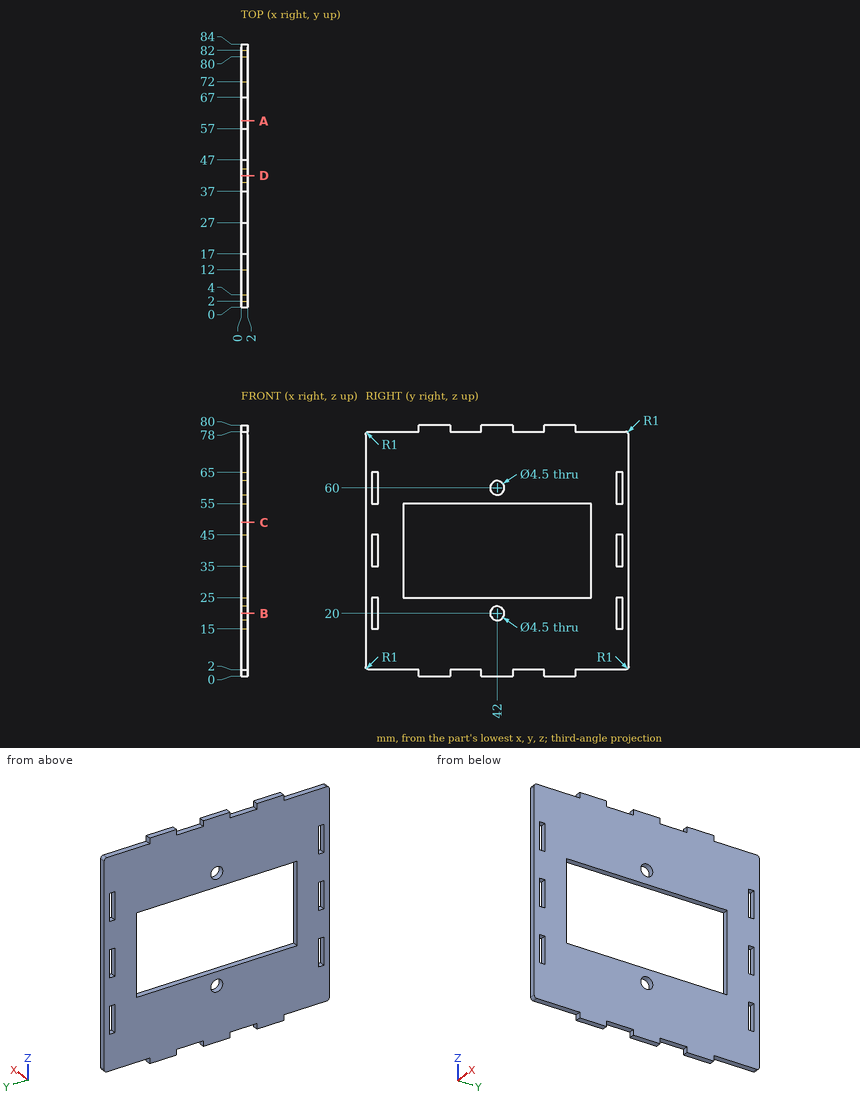
Drawing for the job (mm, zero at the part's lowest x, y, z). Round coordinates to 2 decimals unless told otherwise and drop trailing zeros. Loops run counter-clockwise (first coordinate to the right, second up) from the corner with the lowest first, then second, coordinate; pieces in that order, holes last. Notation, with made-up numbers: (37.25, 65) -> (79.25, 65) arc R16 cw to (79.25, 80) -> close; hole circle Ø4 at (-40, 6). An arc over 180 degrees is marked (long way). Use one line per item in the form item = value. Start each with the question number.
Item 1: Drop flat-ended pins along their axis: pin 1 Ø0.6 at (x, z) = (0.5, 79) entering from -Y; pin 2 Ø1 at (x, z) = (1, 1) entering from +Y. Give the stop position or say it passes through.
Item 2: Band-saw the part on D-D (y = 42). List the corners of the cut face in (x, z), plus the area to 3 significant figures.
Item 3: Drill centre lines: line 1 along Y through (x, z) = (1.4, 62.5); line 2 along Z through (x, y) = (1.5, 42); line 3 along Z through (x, y) = (1.05, 54). Where is each one in solid material? Low to high.
Item 4: Band-saw the part on C-C (z = 49). List the corners of the cut face in (x, y).
Item 5: Band-saw the part on A-A (y = 59.5). List the corners of the cut face in (x, z).
Item 6: Band-saw the part on B-B (z = 20). List the corners of the cut face in (x, y), plus the area to 3 significant figures.
Data:
q1.pin_1 = 17
q1.pin_2 = 67
q2.outline = (0, 0) -> (2, 0) -> (2, 17.75) -> (0, 17.75) -> close; (0, 22.25) -> (2, 22.25) -> (2, 25) -> (0, 25) -> close; (0, 55) -> (2, 55) -> (2, 57.75) -> (0, 57.75) -> close; (0, 62.25) -> (2, 62.25) -> (2, 80) -> (0, 80) -> close
q2.area = 82.0 mm^2
q3.line_1 = 0 to 2, 4 to 80, 82 to 84
q3.line_2 = 0 to 17.75, 22.25 to 25, 55 to 57.75, 62.25 to 80
q3.line_3 = 2 to 25, 55 to 78
q4.outline = (0, 0) -> (2, 0) -> (2, 12) -> (0, 12) -> close; (0, 72) -> (2, 72) -> (2, 84) -> (0, 84) -> close
q5.outline = (0, 0) -> (2, 0) -> (2, 25) -> (0, 25) -> close; (0, 55) -> (2, 55) -> (2, 80) -> (0, 80) -> close
q6.outline = (0, 0) -> (2, 0) -> (2, 2) -> (0, 2) -> close; (0, 4) -> (2, 4) -> (2, 39.75) -> (0, 39.75) -> close; (0, 44.25) -> (2, 44.25) -> (2, 80) -> (0, 80) -> close; (0, 82) -> (2, 82) -> (2, 84) -> (0, 84) -> close
q6.area = 151 mm^2
